Could you check a few things on this drawing? It's one solid part, dimensions in mm from its lowest x, y, z. Round coordinates to 2 decimals unless told otherwise and drop trailing zeros. Write each loop counter-clockwise with the first axis right and the second up, starting at its lowest first coordinate (ties: lowest second). Pieces come first, ordered by that corner, then holes. Notation, with made-up numbers: (-11.5, 70.25) - (17.5, 70.25) arc R25 ccw to (17.5, 82.25) - close; hole circle Ø4 at (69.5, 63). An arc over 180 degrees is marked (long way). Put each result on its own line as item: value.
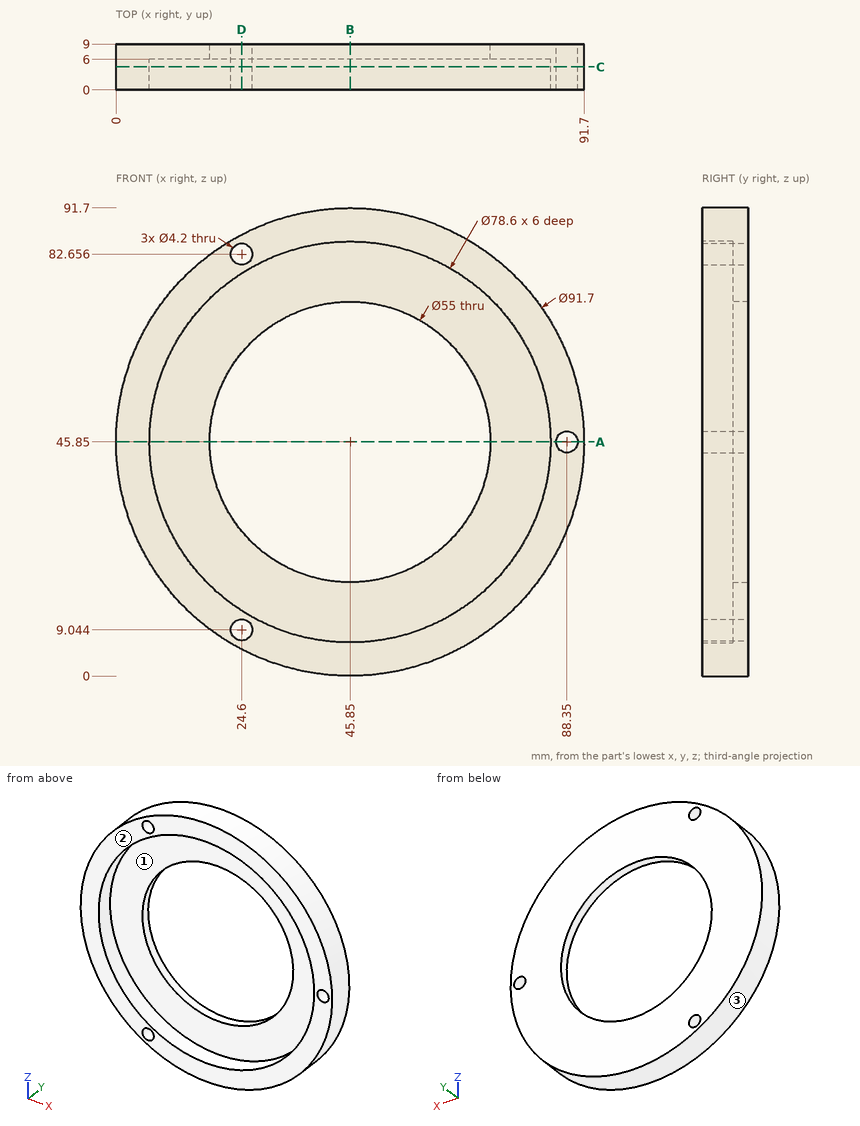
(1) Imagine slicing it at B-B, the plane x = 45.85. List the corners of the cut face in (y, z) for me, then the cut area to 3 significant figures.
Values found:
outline: (0, 0) - (9, 0) - (9, 18.35) - (6, 18.35) - (6, 6.55) - (0, 6.55) - close; (0, 85.15) - (6, 85.15) - (6, 73.35) - (9, 73.35) - (9, 91.7) - (0, 91.7) - close
area: 189 mm^2
(2) Imagine slicing it at D-D, the plane x = 24.6. List the corners of the cut face in (y, z) for me, then the cut area to 3 significant figures.
Values found:
outline: (0, 5.22) - (9, 5.22) - (9, 6.94) - (0, 6.94) - close; (0, 11.14) - (9, 11.14) - (9, 28.39) - (6, 28.39) - (6, 12.79) - (0, 12.79) - close; (0, 78.91) - (6, 78.91) - (6, 63.31) - (9, 63.31) - (9, 80.56) - (0, 80.56) - close; (0, 84.76) - (9, 84.76) - (9, 86.48) - (0, 86.48) - close
area: 154 mm^2
(3) Imagine slicing it at C-C, the plane y = 4.5. List the corners of the cut face in (x, z) for me, then the cut area to 3 significant figures.
Values found:
outline: circle Ø91.7 at (45.85, 45.85); hole circle Ø78.6 at (45.85, 45.85); hole circle Ø4.2 at (24.6, 9.04); hole circle Ø4.2 at (24.6, 82.66); hole circle Ø4.2 at (88.35, 45.85)
area: 1,710 mm^2
(4) Imagine slicing it at A-A, the plane z = 45.85. List the corners of the cut face in (x, y) for me.
Values found:
outline: (0, 0) - (6.55, 0) - (6.55, 6) - (18.35, 6) - (18.35, 9) - (0, 9) - close; (73.35, 6) - (85.15, 6) - (85.15, 0) - (86.25, 0) - (86.25, 9) - (73.35, 9) - close; (90.45, 0) - (91.7, 0) - (91.7, 9) - (90.45, 9) - close
(5) If we mould it in two halves opening along Z, with no side actions, what happens to the marked faces 1, 2 and 3? For each: pulls with the +Z half, pulls with the -Z half, needs draft (parallel to the pull), parting line crosses it, or undercut.
Values found:
face 1: undercut
face 2: needs draft
face 3: parting line crosses it
(6) I'm going to push flat-ended pins straight in: pin 1 (4 mm diameter, centred on y = 4, z = 39, fed in from -X); pin 2 (5 mm diameter, centred on y = 5, z = 69, fed in from -X); pin 3 (1.5 mm diameter, centred on x = 75, z = 33, fed in from -Y). Where does each tip first touch, or does it pass through?
Values found:
pin 1: stops at x = 0.26
pin 2: stops at x = 4.91
pin 3: stops at y = 6
(7) Please list where these lines run through material, in increasing order: probe 1 along X at (y, z) = (7.35, 45.85); probe 2 along X at (y, z) = (4.55, 45.85); probe 3 along Z at (x, y) = (44.5, 3.75). Write a range as from..to.
Values found:
probe 1: x = 0..18.35, 73.35..86.25, 90.45..91.7
probe 2: x = 0..6.55, 85.15..86.25, 90.45..91.7
probe 3: z = 0.02..6.57, 85.13..91.68
